from build123d import *

# Parameters (mm, degrees)
MODEL_R                 = 1.5
SALIENTE_EXTRUIR1_DEPTH = 3


with BuildPart() as part:
    # Model → Saliente-Extruir1 (new body)
    with BuildSketch(Plane.XY):
        with BuildLine():
            Line((256.429131311, 228.742243614), (346.429131311, 228.742243614))
            ThreePointArc((346.429131311, 228.742243614), (349.611111826, 227.424224129), (350.929131311, 224.242243614))
            Line((350.929131311, 224.242243614), (350.929131311, 215.242243614))
            ThreePointArc((350.929131311, 215.242243614), (349.611111826, 212.060263099), (346.429131311, 210.742243614))
            Line((346.429131311, 210.742243614), (256.429131311, 210.742243614))
            ThreePointArc((256.429131311, 210.742243614), (253.247150795, 212.060263099), (251.929131311, 215.242243614))
            Line((251.929131311, 215.242243614), (251.929131311, 224.242243614))
            ThreePointArc((251.929131311, 224.242243614), (253.247150795, 227.424224129), (256.429131311, 228.742243614))
        make_face()
        with Locations((310.429131311, 224.242243614)):
            Circle(MODEL_R, mode=Mode.SUBTRACT)
        with Locations((292.429131311, 224.242243614)):
            Circle(MODEL_R, mode=Mode.SUBTRACT)
        with Locations((301.429131311, 224.242243614)):
            Circle(MODEL_R, mode=Mode.SUBTRACT)
        with Locations((337.429131311, 215.242243614)):
            Circle(MODEL_R, mode=Mode.SUBTRACT)
        with Locations((319.429131311, 215.242243614)):
            Circle(MODEL_R, mode=Mode.SUBTRACT)
        with Locations((328.429131311, 215.242243614)):
            Circle(MODEL_R, mode=Mode.SUBTRACT)
        with Locations((310.429131311, 215.242243614)):
            Circle(MODEL_R, mode=Mode.SUBTRACT)
        with Locations((292.429131311, 215.242243614)):
            Circle(MODEL_R, mode=Mode.SUBTRACT)
        with Locations((301.429131311, 215.242243614)):
            Circle(MODEL_R, mode=Mode.SUBTRACT)
        with Locations((274.429131311, 215.242243614)):
            Circle(MODEL_R, mode=Mode.SUBTRACT)
        with Locations((283.429131311, 215.242243614)):
            Circle(MODEL_R, mode=Mode.SUBTRACT)
        with Locations((265.429131311, 215.242243614)):
            Circle(MODEL_R, mode=Mode.SUBTRACT)
        with Locations((256.429131311, 215.242243614)):
            Circle(MODEL_R, mode=Mode.SUBTRACT)
        with Locations((346.429131311, 215.242243614)):
            Circle(MODEL_R, mode=Mode.SUBTRACT)
        with BuildLine():
            Line((256.429131311, 225.742243614), (283.429131311, 225.742243614))
            ThreePointArc((283.429131311, 225.742243614), (284.929131311, 224.242243614), (283.429131311, 222.742243614))
            Line((283.429131311, 222.742243614), (256.429131311, 222.742243614))
            ThreePointArc((256.429131311, 222.742243614), (254.929131311, 224.242243614), (256.429131311, 225.742243614))
        make_face(mode=Mode.SUBTRACT)
        with BuildLine():
            Line((319.429131311, 225.742243614), (346.429131311, 225.742243614))
            ThreePointArc((346.429131311, 225.742243614), (347.929131311, 224.242243614), (346.429131311, 222.742243614))
            Line((346.429131311, 222.742243614), (319.429131311, 222.742243614))
            ThreePointArc((319.429131311, 222.742243614), (317.929131311, 224.242243614), (319.429131311, 225.742243614))
        make_face(mode=Mode.SUBTRACT)
    extrude(amount=SALIENTE_EXTRUIR1_DEPTH)


solid = part.part
Here's how the part is built. I have some questions about the finished solid (model axes, mm). A direction names the side the tool comes from. Round coordinates to 2 decimals unless told otherwise and drop trailing zeros. Loops run counter-clockwise (first coordinate to the right, second up) from the corner with the lowest first, then second, coordinate; pieces in that order, holes last.
1. If we section it at C-C on x = 261.5: Write out the boundary of the cut face in (y, z), plus the area to 3 significant figures.
Answer list:
outline: (210.74, 0) - (222.74, 0) - (222.74, 3) - (210.74, 3) - close; (225.74, 0) - (228.74, 0) - (228.74, 3) - (225.74, 3) - close
area: 45.0 mm2
2. If we section it at B-B on z = 2.5: Count the separate pieces of the cut face and the enclosed holes in it, plus the area to 3 significant figures.
Answer list:
separate pieces: 1
enclosed holes: 16
area: 1,490 mm2
3. For P1, Ø2.5, axis at x = 283.43, y = 215.24, coming from the +Z side; P2, Ø1.5, axis at y = 213.5, z = 2, coming from the -X side, each with a flat end and sliding along its axis, tell me the tip position at first contact or that it passes through.
Answer list:
P1: passes through
P2: stops at x = 252.04
4. We'd pull the mould along X, two halves only. Please class faces 1 (the face through (349.576, 227.459, 1.479)), 2 (the face through (290.93, 224.31, 1.48)), 3 (the face through (251.929, 220, 1)): +X half, -X half, draft (parallel to the pull), parting line (faces both ways), or undercut.
Answer list:
face 1: +X half
face 2: undercut
face 3: -X half
5. Which directions (+Z, -Z, +X, -X, +Y, -Y) give clear straight access to the entire face, cutting with the end or side of a thin tool? Please do faces 4 (the face through (301, 228.742, 1)), 5 (the face through (270, 222.742, 1)).
Answer list:
face 4: +Z, -Z, +X, -X, +Y
face 5: +Z, -Z
6. If I drill on line 1 along X through (y, z) = (224.25, 2.1); line 2 along Y through (x, z) = (269.5, 2.1); line 3 along Y through (x, z) = (275.5, 2.4), over which ranges is the centre line in solid material (lowest first)?
Answer list:
line 1: x = 251.93 to 254.93, 284.93 to 290.93, 293.93 to 299.93, 302.93 to 308.93, 311.93 to 317.93, 347.93 to 350.93
line 2: y = 210.74 to 222.74, 225.74 to 228.74
line 3: y = 210.74 to 214.19, 216.29 to 222.74, 225.74 to 228.74
7. If we section it at A-A on x = 328.5: Write out the boundary of the cut face in (y, z), plus the area to 3 significant figures.
Answer list:
outline: (210.74, 0) - (213.74, 0) - (213.74, 3) - (210.74, 3) - close; (216.74, 0) - (222.74, 0) - (222.74, 3) - (216.74, 3) - close; (225.74, 0) - (228.74, 0) - (228.74, 3) - (225.74, 3) - close
area: 36.0 mm2
